Check sheet for the drawn part. Datum: minimum x, y, z corner. Units: mm. A direction names the side the tool comes from. Coordinates: 2 decimals unless noted, no trailing zeros. Loops run counter-clockwise (first coordinate to the right, second up) from the corner with the lowest first, then second, coordinate; pieces in that order, holes last.
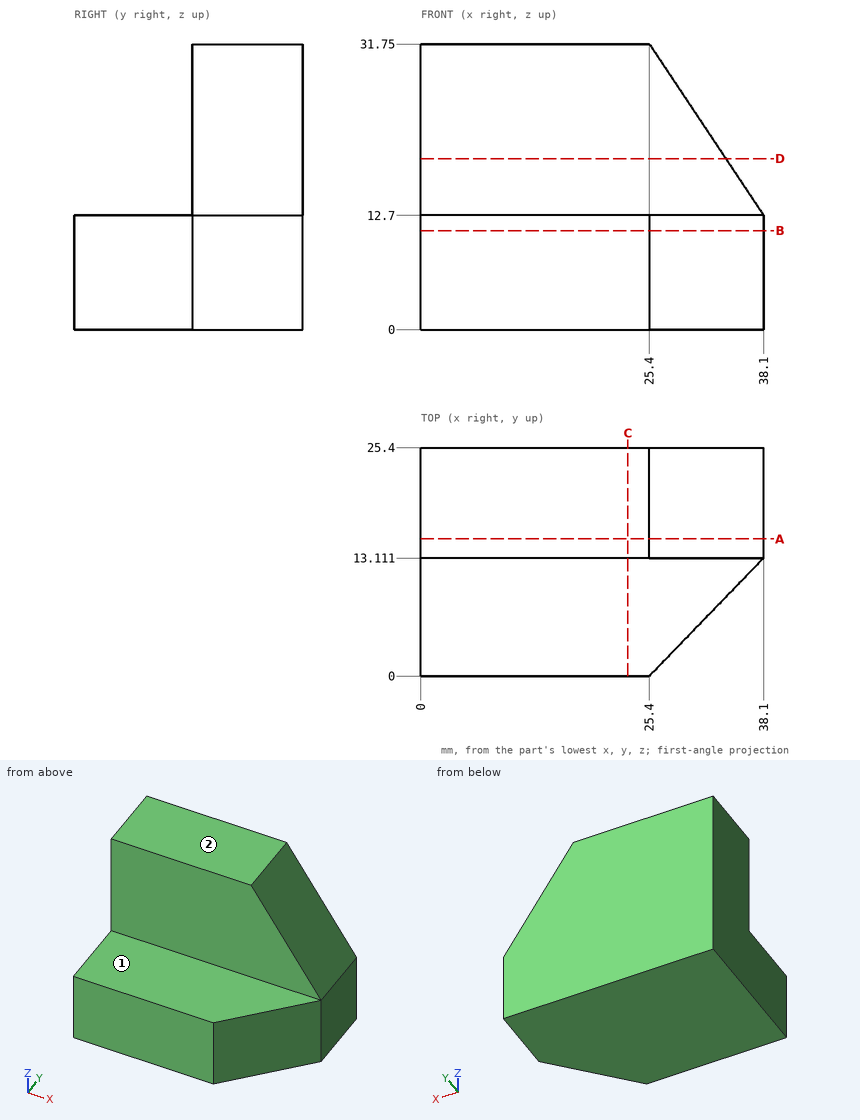
1) Depth check by flat-ended pin: pin 1 (6.5 mm diameter, centred on x = 12, y = 9.5, fed in from +Z); pin 2 (1 mm diameter, centred on y = 19.5, z = 19, fed in from +X); pin 3 (2 mm diameter, centred on x = 30.5, y = 20.5, fed in from +Z). Enter the tip coordinate at first touch or a pass-through.
Answer sheet:
pin 1: stops at z = 12.7
pin 2: stops at x = 34.23
pin 3: stops at z = 25.6
2) Set-up check for the marked faces 1 and 2: record each of +Z, -Z, +X, -X, +Y, -Y from which the full face is reachable in a straight line by a thin tool's end or side.
Answer sheet:
face 1: +Z, +X, -X, -Y
face 2: +Z, +X, -X, +Y, -Y
3) Section check A-A on y = 15.25. Enter the section's corners in (x, z), plus the area to 3 significant figures.
Answer sheet:
outline: (0, 0) - (38.1, 0) - (38.1, 12.7) - (25.4, 31.75) - (0, 31.75) - close
area: 1,090 mm2
4) Scan lines: line 1 (Y direction, x = 27.5, z = 17); line 2 (Z direction, x = 3, y = 12.5); line 3 (Z direction, x = 28, y = 19.5). Record each from-to range of solid material in increasing order.
Answer sheet:
line 1: y = 13.11 to 25.4
line 2: z = 0 to 12.7
line 3: z = 0 to 27.85
5) Section check B-B on z = 11. Enter the section's corners in (x, y).
Answer sheet:
outline: (0, 0) - (25.4, 0) - (38.1, 13.11) - (38.1, 25.4) - (0, 25.4) - close
6) Section check C-C on x = 23. Enter the section's corners in (y, z).
Answer sheet:
outline: (0, 0) - (25.4, 0) - (25.4, 31.75) - (13.11, 31.75) - (13.11, 12.7) - (0, 12.7) - close
7) Section check D-D on z = 19. Enter the section's corners in (x, y), plus the area to 3 significant figures.
Answer sheet:
outline: (0, 13.11) - (33.9, 13.11) - (33.9, 25.4) - (0, 25.4) - close
area: 417 mm2
